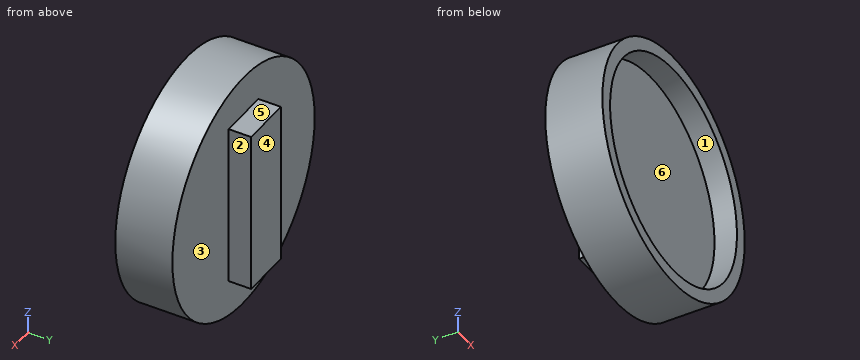
```python
from build123d import *

# Parameters (mm, degrees)
F0_R     = 137.07557
F1_DEPTH = 64.516
F2_R     = 122.229909
F3_DEPTH = 25.4
F4_W     = 57.010982
F4_H     = 185.052022
F5_DEPTH = 25.4


with BuildPart() as f1:
    # F0 (on Front) → F1 (new body)
    with BuildSketch(Plane.XZ):
        Circle(F0_R)
    extrude(amount=F1_DEPTH)

    # F2 (on face) → F3 (cut)
    with BuildSketch(Plane.XZ.offset(64.516)):
        Circle(F2_R)
    extrude(amount=-F3_DEPTH, mode=Mode.SUBTRACT)

    # F4 (on face) → F5 (join)
    with BuildSketch(Plane(origin=(0, 0, 0), x_dir=(-1, 0, 0), z_dir=(0, 1, 0))):
        Rectangle(F4_W, F4_H)
    extrude(amount=F5_DEPTH)


solid = f1.part
```
Here's how the part is built. I have some questions about the finished solid (model axes, mm). Face numbers are marked on the shaded views. A direction names the side the tool comes from. Give positions to 0.01 mm unless a question says otherwise; leave off trailing zeros. Write each loop counter-clockwise with the first axis right and the second up, starting at its lowest first coordinate (ties: lowest second). Pieces come first, ordered by that corner, then holes.
(1) Imagine slicing it at D-D, the plane y = -23. Write out the boundary of the cut face in (x, z).
Output values:
outline: circle Ø274.15 at (0, 0)
(2) Will these pins go through, and if not, where does the flat tip stop? pin 1 (7.5 mm diameter, centred on x = 12, y = 13, fed in from +Z); pin 2 (6 mm diameter, centred on y = -4.5, z = -67.5, fed in from -X); pin 3 (20.5 mm diameter, centred on y = 11, z = -21.5, fed in from -X).
Output values:
pin 1: stops at z = 92.53
pin 2: stops at x = -120.95
pin 3: stops at x = -28.51
(3) Thinking about a two-plate mould opening in X: for the marked faces 1, 2 and 3, which applies, pulls with the +X half, pulls with the -X half, needs draft (parallel to the pull), parting line crosses it, or undercut?
Output values:
face 1: undercut
face 2: pulls with the +X half
face 3: needs draft
(4) Imagine slicing it at B-B, the plane x = 0. Write out the boundary of the cut face in (y, z).
Output values:
outline: (-64.52, -137.08) - (0, -137.08) - (0, -92.53) - (25.4, -92.53) - (25.4, 92.53) - (0, 92.53) - (0, 137.08) - (-64.52, 137.08) - (-64.52, 122.23) - (-39.12, 122.23) - (-39.12, -122.23) - (-64.52, -122.23) - close
(5) If I drill on L1, parallel to Z at x = 0, y = -46.25; L2, parallel to Y at x = -42, z = 120; L3, parallel to Y at x = 70, z = 29.5, over which ranges is the centre line in solid material (lowest first)?
Output values:
L1: z = -137.08 to -122.23, 122.23 to 137.08
L2: y = -64.52 to 0
L3: y = -39.12 to 0
(6) On a 3-axis mill with a long thin cutter (end or side, diameter ignored), from which of +Z, -Z, +X, -X, +Y, -Y can I reach the whole of each face in a straight line? I mean the marked faces 4, 5 and 6. Say none if no direction works.
Output values:
face 4: +Z, -Z, +X, -X, +Y
face 5: +Z, +X, -X, +Y
face 6: -Y
(7) Imagine slicing it at C-C, the plane y = -57.5. Write out the boundary of the cut face in (x, z), and give its area (3 significant figures).
Output values:
outline: circle Ø274.15 at (0, 0); hole circle Ø244.46 at (0, 0)
area: 12,100 mm2
(8) Imagine slicing it at A-A, the plane z = 0. Write out the boundary of the cut face in (x, y), and give its area (3 significant figures).
Output values:
outline: (-137.08, -64.52) - (-122.23, -64.52) - (-122.23, -39.12) - (122.23, -39.12) - (122.23, -64.52) - (137.08, -64.52) - (137.08, 0) - (28.51, 0) - (28.51, 25.4) - (-28.51, 25.4) - (-28.51, 0) - (-137.08, 0) - close
area: 12,900 mm2
